For this review, take the finished solid that the model builds, in its own axes (mm). Face numbers are marked on the shaded views. A direction names the side the tool comes from. Coordinates: 2 decimals unless noted, no trailing zeros. Loops run counter-clockwise (first coordinate to the right, second up) from the corner with the lowest first, then second, coordinate; pieces in that order, holes last.
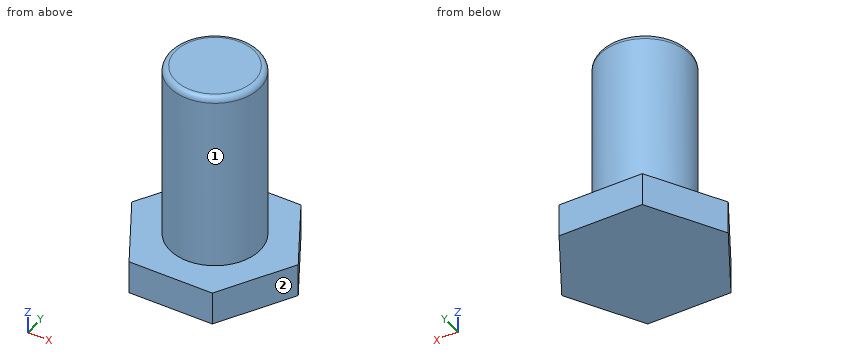
```python
from build123d import *

# Parameters (mm, degrees)
Y_KSEKLIK_EKSTR_ZYON1_DEPTH = 2.95
IZIM3_R                     = 4
Y_KSEKLIK_EKSTR_ZYON2_DEPTH = 16
RADYUS3_R                   = 0.5


with BuildPart() as part:
    # Çizim2 → Yükseklik-Ekstrüzyon1 (new body)
    with BuildSketch(Plane.XY):
        Polygon((3.712848138, 6.376327996), (-3.665637958, 6.403584805), (-7.378486096, 0.02725681), (-3.712848138, -6.376327996), (3.665637958, -6.403584805), (7.378486096, -0.02725681), align=None)
    extrude(amount=Y_KSEKLIK_EKSTR_ZYON1_DEPTH)

    # Çizim3 → Yükseklik-Ekstrüzyon2 (add)
    with BuildSketch(Plane.XY.offset(2.95)):
        Circle(IZIM3_R)
    extrude(amount=Y_KSEKLIK_EKSTR_ZYON2_DEPTH)

    # Radyus3
    radyus3_edges = [part.edges().sort_by_distance(p)[0] for p in [
        (-4, 0, 18.95),
    ]]
    fillet(radyus3_edges, radius=RADYUS3_R)


solid = part.part
```
Q1. Consider section D-D (x = -4.75). State the section outline as (y, z) points, then the cut area to 3 significant figures.
Q2. Consider section B-B (z = 7). State the section outline as (x, y) points, then the cut area to 3 significant figures.
Q3. For pin 1 Ø5 at (x, y) = (-5, 4) entering from -Z; pin 2 Ø4 at (x, z) = (4.5, 13) entering from -Y; pin 3 Ø3 at (x, z) = (-2.5, 12) entering from -Y; pin 4 Ø2 at (x, z) = (3.5, 3) entering from +Y, all flat-tipped, find the tip position at first contact; note any pin that passes through.
Q4. Wall thickness on probe 1 along Z at (x, y) = (-5.5, -0.5); probe 2 along Y at (x, z) = (1.5, 12.5); probe 3 along Y at (x, z) = (0, 14.5): over which ranges is each line inside the solid? List them lowest first.
Q5. Machinability: for the marked faces 1 and 2, which of the approach directions +Z, -Z, +X, -X, +Y, -Y give a long, thin tool a straight path to every point of the face, cutting with its end or side? Answer none if there is none.
Q6. Consider section C-C (y = 4.5). State the section outline as (x, z) points, then the cut area to 3 significant figures.
Q7. Consider section A-A (x = 0). State the section outline as (y, z) points.
Model answer:
1. outline: (-4.56, 0) - (4.54, 0) - (4.54, 2.95) - (-4.56, 2.95) - close
1. area: 26.9 mm2
2. outline: circle Ø8 at (0, 0)
2. area: 50.3 mm2
3. pin 1: stops at z = 0
3. pin 2: stops at y = -3.12
3. pin 3: stops at y = -3.87
3. pin 4: stops at y = 6.38
4. probe 1: z = 0 to 2.95
4. probe 2: y = -3.71 to 3.71
4. probe 3: y = -4 to 4
5. face 1: +Z
5. face 2: +Z, -Z, +X, -Y
6. outline: (-4.77, 0) - (4.79, 0) - (4.79, 2.95) - (-4.77, 2.95) - close
6. area: 28.2 mm2
7. outline: (-6.39, 0) - (6.39, 0) - (6.39, 2.95) - (4, 2.95) - (4, 18.45) arc R0.5 ccw to (3.5, 18.95) - (-3.5, 18.95) arc R0.5 ccw to (-4, 18.45) - (-4, 2.95) - (-6.39, 2.95) - close
